```python
from build123d import *

# Parameters (mm, degrees)
SKETCH3_R                  = 3.2385
BOSS_EXTRUDE1_DEPTH        = 50.8
FILLET1_R                  = 0.254
BOSS_EXTRUDE2_DEPTH        = 38.1
F_8_0_199_DIAMETER_HOLE1_D = 5.0546
LPATTERN1_COUNT            = 2
LPATTERN1_PITCH            = 22.86


with BuildPart() as part:
    # Sketch3 → Boss-Extrude1 (new body, symmetric)
    with BuildSketch(Plane.XY):
        with BuildLine():
            Line((-11.049, 12.7), (-3.302, 12.7))
            Line((-3.302, 12.7), (-3.302, 10.328863887))
            Line((-3.302, 10.328863887), (-6.985, 10.328863887))
            ThreePointArc((-6.985, 10.328863887), (-7.454330803, 10.01526707), (-7.344210245, 9.461653642))
            Line((-7.344210245, 9.461653642), (-3.452505379, 5.569948776))
            ThreePointArc((-3.452505379, 5.569948776), (-2.628470073, 5.019345987), (-1.656454155, 4.826))
            Line((-1.656454155, 4.826), (1.656454155, 4.826))
            ThreePointArc((1.656454155, 4.826), (2.628470073, 5.019345987), (3.452505379, 5.569948776))
            Line((3.452505379, 5.569948776), (7.344210245, 9.461653642))
            ThreePointArc((7.344210245, 9.461653642), (7.454330803, 10.01526707), (6.985, 10.328863887))
            Line((6.985, 10.328863887), (3.302, 10.328863887))
            Line((3.302, 10.328863887), (3.302, 12.7))
            Line((3.302, 12.7), (11.049, 12.7))
            ThreePointArc((11.049, 12.7), (12.216433296, 12.216433296), (12.7, 11.049))
            Line((12.7, 11.049), (12.7, 1.651))
            ThreePointArc((12.7, 1.651), (12.216433296, 0.483566704), (11.049, 0))
            Line((11.049, 0), (-11.049, 0))
            ThreePointArc((-11.049, 0), (-12.216433296, 0.483566704), (-12.7, 1.651))
            Line((-12.7, 1.651), (-12.7, 11.049))
            ThreePointArc((-12.7, 11.049), (-12.216433296, 12.216433296), (-11.049, 12.7))
        make_face()
        with Locations((8.509, 4.064)):
            Circle(SKETCH3_R, mode=Mode.SUBTRACT)
        with Locations((-8.509, 4.064)):
            Circle(SKETCH3_R, mode=Mode.SUBTRACT)
    extrude(amount=BOSS_EXTRUDE1_DEPTH, both=True)

    # Fillet1
    fillet1_edges = [part.edges().sort_by_distance(p)[0] for p in [
        (-3.302, 12.7, 0),
        (-3.302, 10.328863887, 0),
        (3.302, 10.328863887, 0),
        (3.302, 12.7, 0),
    ]]
    fillet(fillet1_edges, radius=FILLET1_R)

    # Sketch4 → Boss-Extrude2 (add)
    with BuildSketch(Plane(origin=(0, 0, 50.8), x_dir=(-1, 0, 0), z_dir=(0, 0, -1))):
        with BuildLine():
            Line((3.556, 12.7), (-11.049, 12.7))
            ThreePointArc((-11.049, 12.7), (-12.216433296, 12.216433296), (-12.7, 11.049))
            Line((-12.7, 11.049), (-12.7, 1.651))
            ThreePointArc((-12.7, 1.651), (-12.216433296, 0.483566704), (-11.049, 0))
            Line((-11.049, 0), (11.049, 0))
            ThreePointArc((11.049, 0), (12.216433296, 0.483566704), (12.7, 1.651))
            Line((12.7, 1.651), (12.7, 11.049))
            ThreePointArc((12.7, 11.049), (12.216433296, 12.216433296), (11.049, 12.7))
            Line((11.049, 12.7), (3.556, 12.7))
        make_face()
    extrude(amount=-BOSS_EXTRUDE2_DEPTH)

    # #8 (0.199) Diameter Hole1 (through all)
    with Locations(Plane(origin=(12.7, 0, 0), x_dir=(0, 0, -1), z_dir=(1, 0, 0))):
        with Locations((-81.28, 6.35)):
            f_8_0_199_diameter_hole1 = Hole(F_8_0_199_DIAMETER_HOLE1_D / 2)

    # LPattern1: #8 (0.199) Diameter Hole1 ×2
    with Locations(*[(0, 0, -i * LPATTERN1_PITCH) for i in range(1, LPATTERN1_COUNT)]):
        add(f_8_0_199_diameter_hole1, mode=Mode.SUBTRACT)


solid = part.part
```
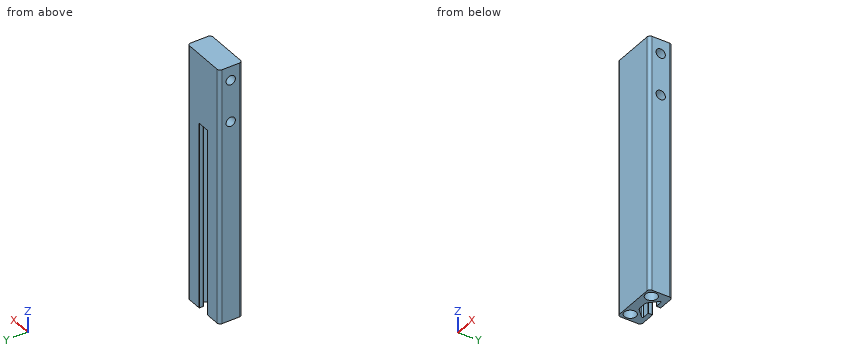
Input: part model. Units: mm. Frame: model coordinates. Coordinates: 2 decimals unless noted, no trailing zeros. Write each loop counter-clockwise with the first axis right and the second up, starting at its lowest first coordinate (ties: lowest second). Pieces come first, ordered by that corner, then holes. Notation, with made-up numbers: M 43.5,89.25 L 82.5,89.25 A18 ccw 82.5,103.25 Z; hole C 59,57.5 d3. An arc over 180 degrees is marked long. Use one line per item in the form item = value.
Q1. First-contact query: pin 1 (1.9 mm diameter, centred on x = -8, y = 5, fed in from -Z); pin 2 (0.9 mm diameter, centred on y = 12, z = -9, fed in from -X); pin 3 (3.5 mm diameter, centred on x = 0.5, z = 23.5, fed in from +Y). Flat tips, straight axial feed; report the tip coordinate or a pass-through.
Answer below:
pin_1 = 50.8
pin_2 = -12.62
pin_3 = 4.9
Q2. Section B-B (z = -30). Count the separate pieces of the cut face and the enclosed holes in it, plus the area to 3 significant figures.
Answer below:
separate_pieces = 1
enclosed_holes = 2
area = 179 mm²
Q3. Material intervals for probe 1 along Z at (x, y) = (1, 6.25); probe 2 along Y at (x, z) = (-6.5, -20.5); probe 3 along X at (y, z) = (4.25, -5.5), sorted ascending. Write a range as from..to.
Answer below:
probe_1 = 50.8..55.89, 60.95..78.75, 83.81..88.9
probe_2 = 0..1.52, 6.6..8.62, 10.33..12.7
probe_3 = -12.7..-11.74, -5.28..5.28, 11.74..12.7
Q4. Section C-C (x = -9.75). Return loops of the section in (y, z), plus the area to 3 significant figures.
Answer below:
outline = M 0,-50.8 L 1.07,-50.8 L 1.07,50.8 L 7.06,50.8 L 7.06,-50.8 L 12.7,-50.8 L 12.7,88.9 L 0,88.9 Z; hole C 6.35,58.42 d5.05; hole C 6.35,81.28 d5.05
area = 1,130 mm²
Q5. Section A-A (z = 81.28). Return loops of the section in (x, y), plus the area to 3 significant figures.
Answer below:
outline = M -12.7,1.65 A1.65 ccw -11.05,0 L 11.05,0 A1.65 ccw 12.7,1.65 L 12.7,3.82 L -12.7,3.82 Z; M -12.7,8.88 L 12.7,8.88 L 12.7,11.05 A1.65 ccw 11.05,12.7 L -11.05,12.7 A1.65 ccw -12.7,11.05 Z
area = 192 mm²
